Geometry: final body of the model. Coordinates: model frame, mm. A direction names the side the tool comes from. Give positions to 0.01 mm unless a question says otherwise; leave off trailing zeros. Write each loop counter-clockwise with the first axis right and the second up, starting at its lowest first coordinate (ties: lowest second). Pieces come first, ordered by that corner, then holes.
from build123d import *

# Parameters (mm, degrees)
SKETCH1_W           = 120
SKETCH1_H           = 36
BOSS_EXTRUDE1_DEPTH = 3.175
CUT_EXTRUDE1_DEPTH  = 63.72224984
SKETCH5_R           = 1
CUT_EXTRUDE2_DEPTH  = 0.5


with BuildPart() as part:
    # Sketch1 → Boss-Extrude1 (new body)
    with BuildSketch(Plane.XY):
        Rectangle(SKETCH1_W, SKETCH1_H)
    extrude(amount=BOSS_EXTRUDE1_DEPTH)

    # Sketch2 → Cut-Extrude1 (cut, through all)
    with BuildSketch(Plane.XY.offset(3.175)):
        with BuildLine():
            Line((20, -15), (-20, -15))
            ThreePointArc((-20, -15), (-35, 0), (-20, 15))
            Line((-20, 15), (20, 15))
            ThreePointArc((20, 15), (35, 0), (20, -15))
        make_face()
    extrude(amount=-CUT_EXTRUDE1_DEPTH, mode=Mode.SUBTRACT)

    # Sketch5 → Cut-Extrude2 (cut)
    with BuildSketch(Plane(origin=(0, 0, 0), x_dir=(-1, 0, 0), z_dir=(0, 0, -1))):
        with Locations((-50, 10)):
            Circle(SKETCH5_R)
        with Locations((-50, -10)):
            Circle(SKETCH5_R)
        with Locations((50, -10)):
            Circle(SKETCH5_R)
        with Locations((50, 10)):
            Circle(SKETCH5_R)
    extrude(amount=-CUT_EXTRUDE2_DEPTH, mode=Mode.SUBTRACT)


solid = part.part
Q1. Section A-A on x = 6. Output: boundary loops of the cut face in (y, z) (3 decimals).
Filled sheet:
outline: (-18, 0) - (-15, 0) - (-15, 3.175) - (-18, 3.175) - close; (15, 0) - (18, 0) - (18, 3.175) - (15, 3.175) - close
Q2. Pull-direction query (X, two-part tool) for faces 1 (the flat face through (60, 0, 2)), 2 (the cylindrical face through (49.046, 10.3, 0.246)), 3 (the flat face through (-1, 18, 2)); classes: released by +X, released by -X, zero draft, split by the parting line, or undercut.
Filled sheet:
face 1: released by +X
face 2: undercut
face 3: zero draft
Q3. Section B-B on z = 1.5. Output: boundary loops of the cut face in (x, y), plus the area to 3 significant figures.
Filled sheet:
outline: (-60, -18) - (60, -18) - (60, 18) - (-60, 18) - close; hole (-20, -15) - (20, -15) arc R15 ccw to (20, 15) - (-20, 15) arc R15 ccw to start
area: 2,410 mm2
Q4. Pin query (flat end, axial travel): P1, Ø0.6, axis at x = 50, y = -10.5, coming from the -Z side. Return the tip coordinate at first contact, or that it passes through.
Filled sheet:
P1: stops at z = 0.5
Q5. Ray query, line 1 along Y through (x, z) = (-50, 0.25); line 2 along Y through (x, z) = (-1, 0.3); line 3 along X through (y, z) = (13.5, 2.4). Return the intervals inside material, ascending.
Filled sheet:
line 1: y = -18 to -11, -9 to 9, 11 to 18
line 2: y = -18 to -15, 15 to 18
line 3: x = -60 to -26.54, 26.54 to 60
Q6. Access query for faces 4 (the flat face through (0, 15, 2)), 5 (the flat face through (50, 10, 0.5)), 6 (the flat face through (-1, -18, 2)). Directions: +Z, -Z, +X, -X, +Y, -Y. A direction counts if a zero-diameter tool reaches every point of the face in a straight line with its end or side. Return the directions, or none.
Filled sheet:
face 4: +Z, -Z
face 5: -Z
face 6: +Z, -Z, +X, -X, -Y
Q7. Section C-C on y = 7.5. Output: boundary loops of the cut face in (x, z) (3 decimals), plus the area to 3 significant figures.
Filled sheet:
outline: (-60, 0) - (-32.99, 0) - (-32.99, 3.175) - (-60, 3.175) - close; (32.99, 0) - (60, 0) - (60, 3.175) - (32.99, 3.175) - close
area: 172 mm2
